The listing builds one solid part. Answer for the finished solid, in the listing's coordinates (mm). A direction names the side the tool comes from. Give positions to 0.01 mm unless a question says otherwise; leave off trailing zeros. Write each loop counter-clockwise with the first axis right and the second up, starting at its lowest first coordinate (ties: lowest second). Pieces come first, ordered by that corner, then holes. Notation, with made-up numbers: (46.25, -22) - (97.25, -22) arc R35 cw to (97.25, 17) - close; hole circle Ø11 at (-37, 19). An arc over 180 degrees is marked (long way). One line per item, written item: value. Start each with the question number.
from build123d import *

# Parameters (mm, degrees)
SKETCH_1_R          = 38
SKETCH_1_R_2        = 2.5
EXTRUDE_1_DEPTH     = 5
SKETCH_5_R          = 2.5
EXTRUDE_3_DEPTH     = 5
CUT_EXTRUDE_1_REACH = 114.375
SKETCH_6_R          = 27.5


with BuildPart() as part:
    # 草图1 → 凸台-拉伸1 (new body)
    with BuildSketch(Plane(origin=(0, 0, 0), x_dir=(1, 0, 0), z_dir=(0, 1, 0))):
        with Locations(Location((0, 0, 0), (0, 0, 270))):
            Circle(SKETCH_1_R)
        with Locations(Location((0, 33, 0), (0, 0, 270))):
            Circle(SKETCH_1_R_2, mode=Mode.SUBTRACT)
    extrude(amount=EXTRUDE_1_DEPTH)

    # 草图5 → 凸台-拉伸3 (add)
    with BuildSketch(Plane(origin=(0, 0, 0), x_dir=(0, 0, -1), z_dir=(1, 0, 0))):
        with BuildLine():
            Line((-25, 30), (-25, 5))
            Line((-25, 5), (25, 5))
            Line((25, 5), (25, 30))
            ThreePointArc((25, 30), (0, 96.618176043), (-25, 30))
        make_face()
        with Locations((0, 91.618176043)):
            Circle(SKETCH_5_R, mode=Mode.SUBTRACT)
    extrude(amount=EXTRUDE_3_DEPTH)

    # 草图6 → 切除-拉伸1 (cut, up to next)
    with BuildSketch(Plane(origin=(5, 0, 0), x_dir=(0, 0, -1), z_dir=(1, 0, 0)), mode=Mode.PRIVATE) as cut_extrude_1_sk1:
        with Locations((0, 58.618176043)):
            Circle(SKETCH_6_R)
    cut_extrude_1_tool1 = extrude(cut_extrude_1_sk1.sketch, amount=-CUT_EXTRUDE_1_REACH, mode=Mode.PRIVATE) & part.part
    add(cut_extrude_1_tool1.solids().sort_by_distance((5, 58.618176, 0))[0], mode=Mode.SUBTRACT)


solid = part.part
Item 1: Find section B-B on y = 62. Determine the outline of the cut face in (x, z), plus the area to 3 significant figures.
Item 2: The mould has two halves that part along X. Classify faces 4 (the flat face through (0, 31, -8)), 5 (the flat face through (5, 31, -8)), 6 (the cylindrical face through (0.1, 2.5, -35.5)): +X half, -X half, draft (parallel to the pull), parting line (faces both ways), or undercut.
Item 3: Find section D-D on z = -33. Determine the outline of the cut face in (x, y).
Item 4: Find section A-A on z = 0. Determine the outline of the cut face in (x, y).
Item 5: Each of these flat-tipped pins is pushed along its axis until it touches: pin 1 Ø4 at (x, y) = (2.5, 14.5) entering from +Z; pin 2 Ø2 at (y, z) = (58, 28) entering from +X; pin 3 Ø4 at (x, y) = (3, 23.5) entering from -Z. Where does it stop, or does it pass through?
Item 6: Straight lines are drawn through the part: line 1 along Y through (x, z) = (26, -23); line 2 along X through (y, z) = (2, -33). For each, find the intervals that lie inside material, in ascending order.
Item 7: For faces 1 (the flat face through (2, 17, -25)), 2 (the flat face through (1, 0, -1)), 3 (the flat face through (2, 18, 25)), determine the directions among +Z, -Z, +X, -X, +Y, -Y from which every point of the face is accessible in a straight line to the end or side of a thin tool.
Item 8: Find section C-C on z = 9. Determine the outline of the cut face in (x, y).
Values:
1. outline: (0, -37.85) - (5, -37.85) - (5, -27.29) - (0, -27.29) - close; (0, 27.29) - (5, 27.29) - (5, 37.85) - (0, 37.85) - close
1. area: 106 mm^2
2. face 4: -X half
2. face 5: +X half
2. face 6: undercut
3. outline: (-18.84, 0) - (-2.5, 0) - (-2.5, 5) - (-18.84, 5) - close; (0, 39.78) - (5, 39.78) - (5, 77.46) - (0, 77.46) - close; (2.5, 0) - (18.84, 0) - (18.84, 5) - (2.5, 5) - close
4. outline: (-38, 0) - (38, 0) - (38, 5) - (5, 5) - (5, 31.12) - (0, 31.12) - (0, 5) - (-38, 5) - close; (0, 86.12) - (5, 86.12) - (5, 89.12) - (0, 89.12) - close; (0, 94.12) - (5, 94.12) - (5, 96.62) - (0, 96.62) - close
5. pin 1: z = 25
5. pin 2: x = 5
5. pin 3: z = -25
6. line 1: 0 to 5
6. line 2: -18.84 to -2.5, 2.5 to 18.84
7. face 1: -Z, +X, -X
7. face 2: +Z, -Z, +X, -X, -Y
7. face 3: +Z, +X, -X
8. outline: (-36.92, 0) - (36.92, 0) - (36.92, 5) - (5, 5) - (5, 32.63) - (0, 32.63) - (0, 5) - (-36.92, 5) - close; (0, 84.6) - (5, 84.6) - (5, 95.54) - (0, 95.54) - close
